For this review, take the finished solid that the model builds, in its own axes (mm). A direction names the side the tool comes from. Round coordinates to 2 decimals unless told otherwise and drop trailing zeros. Write each loop counter-clockwise with the first axis right and the second up, starting at its lowest first coordinate (ties: lowest second). Pieces come first, ordered by that corner, then holes. Notation, with made-up numbers: (26.5, -31.75) -> (53.5, -31.75) arc R14 cw to (53.5, -14.75) -> close; hole circle Ø5 at (3, -5.75). An arc over 180 degrees is marked (long way). Answer as CSV lines item,"result". Start each with the question number.
Item 1: Machinability: for faces 1 (the flat face through (320.865, 107, 18)), 2 (the flat face through (332, 89.55, 18)), 3 (the flat face through (314.865, 79, 18)), which of the approach directions +Z, -Z, +X, -X, +Y, -Y give a long, thin tool a straight path to every point of the face, cutting with its end or side? Answer none if there is none.
Item 2: Wall thickness on probe 1 along Y at (x, z) = (331, 15); probe 2 along X at (y, z) = (106, 31); probe 3 along Y at (x, z) = (326, 20): over which ranges is each line inside the solid? List them lowest first. Write a range as from..to.
Item 3: Take a section at C-C on y = 104.5. Give the boundary of the cut face in (x, z), then the cut area to 3 significant figures.
Item 4: Take a section at D-D on y = 91.5. Give the boundary of the cut face in (x, z), then the cut area to 3 significant figures.
Item 5: Take a section at B-B on z = 11. Give the boundary of the cut face in (x, y).
Item 6: For pin 1 Ø6 at (x, z) = (326, 48) entering from -Y; pin 2 Ø4 at (x, y) = (318.5, 91.5) entering from +Z; pin 3 Ø10 at (x, z) = (311.5, 51.5) entering from +Y, all flat-tipped, find the tip position at first contact; note any pin that passes through.
Item 7: Mouldability with a two-part tool opening along X and no side actions: class faces 4 (the flat face through (309, 107.55, 18)), 5 (the flat face through (320, 105.55, 19)), 6 (the flat face through (304.865, 90.6, 19)) as +X half, -X half, draft (parallel to the pull), parting line (faces both ways), or undercut.
Item 8: Take a section at A-A on z = 20. Count the separate pieces of the cut face and the enclosed holes in it, then the cut area to 3 significant figures.
```python
from build123d import *

# Parameters (mm, degrees)
SKETCH1_W                           = 30
SKETCH1_H                           = 30
BOSS_EXTRUDE1_DEPTH                 = 37.5
SKETCH2_R                           = 6
SKETCH2_R_2                         = 4.025
BOSS_EXTRUDE2_DEPTH                 = 20
CUT_EXTRUDE1_START                  = -10
SKETCH3_R                           = 4.025
CUT_EXTRUDE1_DEPTH                  = 10
SKETCH4_W                           = 6
SKETCH4_H                           = 75
CUT_EXTRUDE2_DEPTH                  = 2
CIRPATTERN1_COUNT                   = 4
SKETCH5_R                           = 2
CUT_EXTRUDE3_DEPTH                  = 126.128763374
SKETCH6_R                           = 2
CUT_EXTRUDE4_DEPTH                  = 339.953272019
M3X0_5_TAPPED_HOLE1_REACH           = 52.721
M3X0_5_TAPPED_HOLE1_BORE_R          = 1.25
M3X0_5_TAPPED_HOLE1_ON_FACE_2_REACH = 60.509
M3X0_5_TAPPED_HOLE1_BORE_2_R        = 1.25


with BuildPart() as part:
    # Sketch1 → Boss-Extrude1 (new body)
    with BuildSketch(Plane.XY):
        with Locations((317.864943501, 92.549790439)):
            Rectangle(SKETCH1_W, SKETCH1_H)
    extrude(amount=BOSS_EXTRUDE1_DEPTH)

    # Sketch2 → Boss-Extrude2 (add)
    with BuildSketch(Plane.XY.offset(37.5)):
        with Locations(Location((317.864943501, 92.549790439, 0), (0, 0, 180))):
            Circle(SKETCH2_R)
        with Locations((317.864943501, 92.549790439)):
            Circle(SKETCH2_R_2, mode=Mode.SUBTRACT)
    extrude(amount=BOSS_EXTRUDE2_DEPTH)

    # Sketch3 → Cut-Extrude1 (cut)
    with BuildSketch(Plane.XY.offset(37.5).offset(CUT_EXTRUDE1_START)):
        with Locations((317.864943501, 92.549790439)):
            Circle(SKETCH3_R)
    extrude(amount=CUT_EXTRUDE1_DEPTH, mode=Mode.SUBTRACT)

    # Sketch4 → Cut-Extrude2 (cut)
    with BuildSketch(Plane.XZ.offset(-77.549790439)):
        with Locations((317.864943501, 0)):
            Rectangle(SKETCH4_W, SKETCH4_H)
    cut_extrude2 = extrude(amount=-CUT_EXTRUDE2_DEPTH, mode=Mode.SUBTRACT)

    # CirPattern1: Cut-Extrude2 ×4 about axis
    cirpattern1_axis = Axis((317.864943501, 92.549790439, 0), (0, 0, 1))
    for i in range(1, CIRPATTERN1_COUNT):
        add(cut_extrude2.rotate(cirpattern1_axis, i * 360 / CIRPATTERN1_COUNT), mode=Mode.SUBTRACT)

    # Sketch5 → Cut-Extrude3 (cut, through all)
    with BuildSketch(Plane(origin=(330.864943501, 0, 0), x_dir=(0, 0, -1), z_dir=(1, 0, 0))):
        with Locations(Location((-20, 92.549790439, 0), (0, 0, 90))):
            Circle(SKETCH5_R)
    extrude(amount=-CUT_EXTRUDE3_DEPTH, mode=Mode.SUBTRACT)

    # Sketch6 → Cut-Extrude4 (cut, through all)
    with BuildSketch(Plane.XZ.offset(-79.549790439)):
        with Locations(Location((317.864943501, 20, 0), (0, 0, 270))):
            Circle(SKETCH6_R)
    extrude(amount=-CUT_EXTRUDE4_DEPTH, mode=Mode.SUBTRACT)

    # M3x0.5 Tapped Hole1 bore (on position points) → M3x0.5 Tapped Hole1 (cut, up to next)
    with BuildSketch(Plane(origin=(317.711998096, 86.551740114, 43.612753669), x_dir=(-0.99967505419, 0.025490900946, 0), z_dir=(-0.025490900946, -0.99967505419, 0)), mode=Mode.PRIVATE) as m3x0_5_tapped_hole1_sk1:
        Circle(M3X0_5_TAPPED_HOLE1_BORE_R)
    m3x0_5_tapped_hole1_tool1 = extrude(m3x0_5_tapped_hole1_sk1.sketch, amount=-M3X0_5_TAPPED_HOLE1_REACH, mode=Mode.PRIVATE) & part.part
    add(m3x0_5_tapped_hole1_tool1.solids().sort_by_distance((317.711998, 86.55174, 43.612754))[0], mode=Mode.SUBTRACT)

    # M3x0.5 Tapped Hole1 bore 2 (on position points) → M3x0.5 Tapped Hole1 on face 2 (cut, up to next)
    with BuildSketch(Plane(origin=(317.668420808, 86.553009734, 52.454806576), x_dir=(-0.99946344332, 0.032754014528, 0), z_dir=(-0.032754014528, -0.99946344332, 0)), mode=Mode.PRIVATE) as m3x0_5_tapped_hole1_on_face_2_sk1:
        Circle(M3X0_5_TAPPED_HOLE1_BORE_2_R)
    m3x0_5_tapped_hole1_on_face_2_tool1 = extrude(m3x0_5_tapped_hole1_on_face_2_sk1.sketch, amount=-M3X0_5_TAPPED_HOLE1_ON_FACE_2_REACH, mode=Mode.PRIVATE) & part.part
    add(m3x0_5_tapped_hole1_on_face_2_tool1.solids().sort_by_distance((317.668421, 86.55301, 52.454807))[0], mode=Mode.SUBTRACT)


solid = part.part
```
Output values:
1,face 1,"+Z, -Z, +Y"
1,face 2,"+Z, -Z, +X"
1,face 3,"+Z, -Z, -Y"
2,probe 1,"y = 77.55..89.55, 95.55..107.55"
2,probe 2,"x = 302.86..314.86, 320.86..332.86"
2,probe 3,"y = 77.55..90.55, 94.55..107.55"
3,outline,"(302.86, 0) -> (332.86, 0) -> (332.86, 37.5) -> (302.86, 37.5) -> close; hole circle Ø4 at (317.86, 20)"
3,area,"1,110 mm^2"
4,outline,"(304.86, 0) -> (330.86, 0) -> (330.86, 18.3) -> (318.91, 18.3) arc R2 cw to (316.82, 18.3) -> (304.86, 18.3) -> close; (304.86, 21.7) -> (316.82, 21.7) arc R2 cw to (318.91, 21.7) -> (330.86, 21.7) -> (330.86, 37.5) -> (323.77, 37.5) -> (323.77, 57.5) -> (321.75, 57.5) -> (321.75, 27.5) -> (313.98, 27.5) -> (313.98, 57.5) -> (311.96, 57.5) -> (311.96, 37.5) -> (304.86, 37.5) -> close"
4,area,"889 mm^2"
5,outline,"(302.86, 77.55) -> (314.86, 77.55) -> (314.86, 79.55) -> (320.86, 79.55) -> (320.86, 77.55) -> (332.86, 77.55) -> (332.86, 89.55) -> (330.86, 89.55) -> (330.86, 95.55) -> (332.86, 95.55) -> (332.86, 107.55) -> (320.86, 107.55) -> (320.86, 105.55) -> (314.86, 105.55) -> (314.86, 107.55) -> (302.86, 107.55) -> (302.86, 95.55) -> (304.86, 95.55) -> (304.86, 89.55) -> (302.86, 89.55) -> close"
6,pin 1,"stops at y = 89.45"
6,pin 2,"stops at z = 27.5"
6,pin 3,"stops at y = 98.39"
7,face 4,"draft"
7,face 5,"undercut"
7,face 6,"-X half"
8,separate pieces,"4"
8,enclosed holes,"0"
8,area,"660 mm^2"
